Build history of the part. All positions in model axes, mm. A direction names the side the tool comes from. Round coordinates to 2 decimals unless told otherwise and drop trailing zeros. Write each loop counter-clockwise with the first axis right and the second up, starting at its lowest first coordinate (ties: lowest second). Pieces come first, ordered by that corner, then holes. Notation, with made-up numbers: M 83,-34.5 L 125,-34.5 A15 ccw 125,-30.5 Z; hole C 79,2 d6. An arc over 180 degrees is marked long. Use a Markdown table: item, result.
from build123d import *

# Parameters (mm, degrees)
SKETCH1_R                  = 50
EXTRUDE1_DEPTH             = 25
EXTRUDE1_DRAFT             = -30
SKETCH2_R                  = 12.5
EXTRUDE2_DEPTH             = 25
SKETCH3_R                  = 8
CUT_EXTRUDE1_DEPTH         = 16
F_11_0_11_DIAMETER_HOLE1_D = 11
CUT_EXTRUDE2_DEPTH         = 76


with BuildPart() as part:
    # Sketch1 → Extrude1 (with draft: the straight prism first)
    with BuildSketch(Plane.XY):
        Circle(SKETCH1_R)
    extrude(amount=-EXTRUDE1_DEPTH)
    # Extrude1: the draft: its side faces are tilted about the plane it starts from
    extrude1_sides = [part.faces().sort_by_distance(p)[0] for p in [
        (-50, 0, -12.5),
    ]]
    draft(extrude1_sides, Plane.XY, EXTRUDE1_DRAFT)

    # Sketch2 → Extrude2 (add)
    with BuildSketch(Plane(origin=(0, 0, -25), x_dir=(-1, 0, 0), z_dir=(0, 0, -1))):
        with Locations(Location((0, 0, 0), (0, 0, 180))):
            Circle(SKETCH2_R)
    extrude(amount=EXTRUDE2_DEPTH)

    # Sketch3 → Cut-Extrude1 (cut)
    with BuildSketch(Plane(origin=(0, 0, -50), x_dir=(-1, 0, 0), z_dir=(0, 0, -1))):
        Circle(SKETCH3_R)
    extrude(amount=-CUT_EXTRUDE1_DEPTH, mode=Mode.SUBTRACT)

    # Ø11.0 (11) Diameter Hole1 (through all)
    with Locations(Plane.XY):
        with Locations((0, 0)):
            Hole(F_11_0_11_DIAMETER_HOLE1_D / 2)

    # Sketch7 → Cut-Extrude2 (cut, through all)
    with BuildSketch(Plane(origin=(0, 0, -25), x_dir=(-1, 0, 0), z_dir=(0, 0, -1))):
        Polygon((-55, 42), (60, 42), (60, -42), (-55, -42), (-55, -67), (80, -67), (80, 67), (-55, 67), align=None)
    extrude(amount=-CUT_EXTRUDE2_DEPTH, mode=Mode.SUBTRACT)


solid = part.part
Q1. Two-plate mould, pull along X, no slides. Class faces 3 (the conical face through (19.606, 30.751, -23.436)), 4 (the flat face through (-1.7, 5.4, -34)), 5 (the flat face through (-0.2, 8.2, -50)): +X half, -X half, draft (parallel to the pull), parting line (faces both ways), or undercut.
Response values:
| item | result |
|---|---|
| face 3 | parting line |
| face 4 | undercut |
| face 5 | draft |
Q2. Drop flat-ended pins along their axis: P1, Ø21.5, axis at x = -7, y = 14.5, coming from the -Z side; P2, Ø4, axis at y = -30.5, z = -16.5, coming from the +X side; P3, Ø5, axis at x = -16.5, z = -12.5, coming from the +Y side; P4, Ø1.5, axis at x = 0.5, z = -38, coming from the +Y side. Give the stop position or say it passes through.
Response values:
| item | result |
|---|---|
| P1 | stops at z = -50 |
| P2 | stops at x = 29.32 |
| P3 | stops at y = 41.31 |
| P4 | stops at y = 12.5 |
Q3. Which spindle directions (+Z, -Z, +X, -X, +Y, -Y) get a long thin tool onto all of the face, cutting with end or side? Do faces 1 (the cylindrical face through (1.73, -7.81, -42.11)), 2 (the cylindrical face through (1.19, -5.37, -17.24)). Say none if no direction does.
Response values:
| item | result |
|---|---|
| face 1 | -Z |
| face 2 | +Z, -Z |
Q4. Cut at A-A on x = 0. Give the cut face in (y, z), and give its area (3 significant figures).
Response values:
| item | result |
|---|---|
| outline | M -42,-13.86 L -35.57,-25 L -12.5,-25 L -12.5,-50 L -8,-50 L -8,-34 L -5.5,-34 L -5.5,0 L -42,0 Z; M 5.5,-34 L 8,-34 L 8,-50 L 12.5,-50 L 12.5,-25 L 35.57,-25 L 42,-13.86 L 42,0 L 5.5,0 Z |
| area | 2,020 mm2 |
Q5. Cut at D-D on z = -27. Give the cut face in (x, y).
Response values:
| item | result |
|---|---|
| outline | C 0,0 d25; hole C 0,0 d11 |
Q6. Cut at C-C on z = -37. Give the cut face in (x, y).
Response values:
| item | result |
|---|---|
| outline | C 0,0 d25; hole C 0,0 d16 |
Q7. Drill centre lines: L1, parallel to Y at x = 0, z = -8; L2, parallel to X at y = 0.5, z = -31.5; L3, parallel to Z at x = 9, y = 24. Where is each one in solid material? Low to high.
Response values:
| item | result |
|---|---|
| L1 | y = -42 to -5.5, 5.5 to 42 |
| L2 | x = -12.49 to -5.48, 5.48 to 12.49 |
| L3 | z = -25 to 0 |
Q8. Cut at B-B on y = 0. Give the cut face in (x, z).
Response values:
| item | result |
|---|---|
| outline | M -50,0 L -35.57,-25 L -12.5,-25 L -12.5,-50 L -8,-50 L -8,-34 L -5.5,-34 L -5.5,0 Z; M 5.5,-34 L 8,-34 L 8,-50 L 12.5,-50 L 12.5,-25 L 35.57,-25 L 50,0 L 5.5,0 Z |
